Part model, mm, in its own coordinate system. A direction names the side the tool comes from. Coordinates: 2 decimals unless noted, no trailing zeros. Write each loop counter-clockwise with the first axis right and the second up, starting at its lowest first coordinate (ties: lowest second). Pieces come first, ordered by that corner, then holes. Notation, with made-up numbers: M 82.5,74 L 128.5,74 A23 cw 128.5,103 Z; hole C 48.5,7 d7. An arc over 180 degrees is marked long. Use a Markdown table: item, result. Add a question column.
Q1. Wall check: L1, parallel to Y at x = 0, z = 34; L2, parallel to Z at x = 6.75, y = 4; L3, parallel to X at y = 0.5, z = -4. Give the ranges that are in metal, low to high. Write a range as from..to.
Q2. Slice it at A-A on x = 0. Write the cut outline in (y, z), then the cut area to 3 significant figures.
Q3. Slice it at C-C on z = 64.5. Write the cut outline in (x, y).
Q4. Tool access for faces 1 (the flat face through (5, 0, 0)), 2 (the flat face through (2.1, 2.1, -10)), 3 (the cylindrical face through (2.58, -4.05, 104.93)): list every direction of +Z, -Z, +X, -X, +Y, -Y with a clear straight run to the whole face (end or side of a thin tool).
Q5. Pin check, flat tips, straight feed: pin 1 Ø1 at (x, z) = (2, 53) entering from +Y; pin 2 Ø1.5 at (x, z) = (3.5, 84.5) entering from -Y. Stop position of each tip, or through.
from build123d import *

# Parameters (mm, degrees)
SKETCH_R          = 8
PAD_DEPTH         = 100
SKETCH001_R       = 4.8
PAD001_DEPTH      = 10
PAD001_DEPTH_BACK = 110
SKETCH002_R       = 2.75
POCKET_DEPTH      = 120.001


with BuildPart() as part:
    # Sketch → Pad (new body)
    with BuildSketch(Plane.XY):
        Circle(SKETCH_R)
    extrude(amount=PAD_DEPTH)

    # Sketch001 → Pad001 (new body, two sides)
    with BuildSketch(Plane(origin=(0, 0, 0), x_dir=(1, 0, 0), z_dir=(0, 0, -1))) as pad001_sk:
        Circle(SKETCH001_R)
    extrude(amount=PAD001_DEPTH)
    extrude(pad001_sk.sketch, amount=-PAD001_DEPTH_BACK)

    # Sketch002 → Pocket (cut, through all)
    with BuildSketch(Plane(origin=(0, 0, -10), x_dir=(1, 0, 0), z_dir=(0, 0, -1))):
        Circle(SKETCH002_R)
    extrude(amount=-POCKET_DEPTH, mode=Mode.SUBTRACT)


solid = part.part
Recorded:
| question | item | result |
|---|---|---|
| 1 | L1 | -8..-2.75, 2.75..8 |
| 1 | L2 | 0..100 |
| 1 | L3 | -4.77..-2.7, 2.7..4.77 |
| 2 | outline | M -8,0 L -4.8,0 L -4.8,-10 L -2.75,-10 L -2.75,110 L -4.8,110 L -4.8,100 L -8,100 Z; M 2.75,-10 L 4.8,-10 L 4.8,0 L 8,0 L 8,100 L 4.8,100 L 4.8,110 L 2.75,110 Z |
| 2 | area | 1,130 mm² |
| 3 | outline | C 0,0 d16; hole C 0,0 d5.5 |
| 4 | face 1 | -Z |
| 4 | face 2 | -Z, +X, -X, +Y, -Y |
| 4 | face 3 | +Z |
| 5 | pin 1 | y = 7.86 |
| 5 | pin 2 | y = -7.51 |
